Work out the finished part from the listing and answer in its coordinate system (mm). A direction names the side the tool comes from. Round coordinates to 2 decimals unless told otherwise and drop trailing zeros. Loops run counter-clockwise (first coordinate to the right, second up) from the corner with the lowest first, then second, coordinate; pieces in that order, holes last. Notation, with made-up numbers: (58.25, -27.5) -> (114.25, -27.5) arc R16 ccw to (114.25, -3.5) -> close; hole circle Ø4 at (84.5, 71). An arc over 180 degrees is marked (long way). Write item = value, one per line. Start each with the question number.
```python
from build123d import *

# Parameters (mm, degrees)
SKETCH_W        = 69
SKETCH_H        = 43
PAD_DEPTH       = 23
THICKNESS_T     = 1.5
SKETCH001_R     = 1.5
HOLE_DEPTH      = 2.098709
HOLE_TIPS_R     = 1.5
POCKET_DEPTH    = 5
SKETCH003_W     = 8
SKETCH003_H     = 8
PAD001_DEPTH    = 5
SKETCH007_R     = 2.5
POCKET003_DEPTH = 7
SKETCH008_R     = 2.5
POCKET004_DEPTH = 7
SKETCH009_R     = 2.5
POCKET005_DEPTH = 7
SKETCH010_R     = 2.5
POCKET006_DEPTH = 7
POCKET007_DEPTH = 3
FILLET_R        = 1
FILLET001_R     = 1


with BuildPart() as part:
    # Sketch → Pad (new body)
    with BuildSketch(Plane.XY):
        Rectangle(SKETCH_W, SKETCH_H)
    extrude(amount=PAD_DEPTH)

    # Thickness
    thickness_openings = [part.faces().sort_by_distance(p)[0] for p in [
        (0, 0, 23),
    ]]
    offset(amount=THICKNESS_T, openings=thickness_openings)

    # Sketch001 (on Face10 of Thickness) → Hole (cut)
    with BuildSketch(Plane.YZ.offset(36)):
        with Locations((0, 9)):
            Circle(SKETCH001_R)
    extrude(amount=-HOLE_DEPTH, mode=Mode.SUBTRACT)

    # Hole tips → Hole tip 1 section 0
    with BuildSketch(Plane.YZ.offset(33.901291), mode=Mode.PRIVATE) as hole_tip_1_s0:
        with Locations((0, 9)):
            Circle(HOLE_TIPS_R)
    loft([hole_tip_1_s0.sketch, Vertex(33, 0, 9)], mode=Mode.SUBTRACT)

    # Sketch002 (on Face9 of Hole) → Pocket (cut)
    with BuildSketch(Plane(origin=(-36, 0, 0), x_dir=(0, -1, 0), z_dir=(-1, 0, 0))):
        with BuildLine():
            ThreePointArc((-5, 15), (-8, 12), (-5, 9))
            Line((-5, 9), (5, 9))
            ThreePointArc((5, 9), (8, 12), (5, 15))
            Line((-5, 15), (5, 15))
        make_face()
    extrude(amount=-POCKET_DEPTH, mode=Mode.SUBTRACT)

    # Sketch003 (on Face4 of Pocket) → Pad001 (join)
    with BuildSketch(Plane.XY):
        with Locations((-28.95, 15.925)):
            Rectangle(SKETCH003_W, SKETCH003_H)
        with Locations((28.95, 15.925)):
            Rectangle(SKETCH003_W, SKETCH003_H)
        with Locations((-28.95, -15.925)):
            Rectangle(SKETCH003_W, SKETCH003_H)
        with Locations((28.95, -15.925)):
            Rectangle(SKETCH003_W, SKETCH003_H)
    extrude(amount=PAD001_DEPTH)

    # Sketch007 (on Face39 of Pad001) → Pocket003 (cut)
    with BuildSketch(Plane.XY.offset(5)):
        with Locations((-28.95, 15.925)):
            Circle(SKETCH007_R)
    extrude(amount=-POCKET003_DEPTH, mode=Mode.SUBTRACT)

    # Sketch008 (on Face38 of Pocket003) → Pocket004 (cut)
    with BuildSketch(Plane.XY.offset(5)):
        with Locations((28.95, 15.925)):
            Circle(SKETCH008_R)
    extrude(amount=-POCKET004_DEPTH, mode=Mode.SUBTRACT)

    # Sketch009 (on Face37 of Pocket004) → Pocket005 (cut)
    with BuildSketch(Plane.XY.offset(5)):
        with Locations((-28.95, -15.925)):
            Circle(SKETCH009_R)
    extrude(amount=-POCKET005_DEPTH, mode=Mode.SUBTRACT)

    # Sketch010 (on Face36 of Pocket005) → Pocket006 (cut)
    with BuildSketch(Plane.XY.offset(5)):
        with Locations((28.95, -15.925)):
            Circle(SKETCH010_R)
    extrude(amount=-POCKET006_DEPTH, mode=Mode.SUBTRACT)

    # Sketch011 (on Face52 of Pocket006) → Pocket007 (cut)
    with BuildSketch(Plane(origin=(0, 0, -1.5), x_dir=(1, 0, 0), z_dir=(0, 0, -1))):
        Polygon((-25.145774, 17.161068), (-28.95, 19.925), (-32.754226, 17.161068), (-31.301141, 12.688932), (-26.598859, 12.688932), align=None)
        Polygon((26.598859, 12.688932), (31.301141, 12.688932), (32.754226, 17.161068), (28.95, 19.925), (25.145774, 17.161068), align=None)
        Polygon((-26.598859, -12.688932), (-31.301141, -12.688932), (-32.754226, -17.161068), (-28.95, -19.925), (-25.145774, -17.161068), align=None)
        Polygon((26.598859, -12.688932), (25.145774, -17.161068), (28.95, -19.925), (32.754226, -17.161068), (31.301141, -12.688932), align=None)
    extrude(amount=-POCKET007_DEPTH, mode=Mode.SUBTRACT)

    # Fillet
    fillet_edges = [part.edges().sort_by_distance(p)[0] for p in [
        (34.5, 0, 10.5),
    ]]
    fillet(fillet_edges, radius=FILLET_R)

    # Fillet001
    fillet001_edges = [part.edges().sort_by_distance(p)[0] for p in [
        (-36, 0, 0),
        (-36, -21.5, 11.5),
        (-36, 21.5, 11.5),
        (-36, 0, 23),
        (-36, 8, 12),
        (-36, 0, 9),
        (-36, -8, 12),
        (-36, 0, 15),
    ]]
    fillet(fillet001_edges, radius=FILLET001_R)


solid = part.part
```
Item 1: Section B-B (y = -4) is taken. Determine the outline of the cut face in (x, z), then the cut area to 3 significant figures.
Item 2: Find the intervals of material crossed by line 1 along X through (y, z) = (19, 2); line 2 along Y through (x, z) = (-28.95, 2.75) (3 decimals); line 3 along X through (y, z) = (16.5, 15), in increasing order. Write a range as [from, to].
Item 3: The mould has two halves that part along X. Classify faces 4 (the flat face through (0, -21.5, 11)), 5 (the cylindrical face through (35.754, -0.325, 7.536)), 6 (the cylindrical face through (35.57, 22.55, 11.15)): pulls with the +X half, pulls with the -X half, needs draft (parallel to the pull), parting line crosses it, or undercut.
Item 4: Section A-A (z = 19.5) is taken. Determine the outline of the cut face in (x, y).
Item 5: Section C-C (x = -18.5) is taken. Determine the outline of the cut face in (y, z).
Item 6: A flat-ended cylindrical pin translates along its axis: pin 1 (10 mm diameter, centred on x = 24, y = -13, fed in from +Z). Find the tip coordinate at first contact, or state that the pin passes through.
Item 7: A tool of negligible diameter and unlimited length cuts with its end or side. For faces 1 (the cylindrical face through (35.57, 0.3, -1.05)), 2 (the flat face through (-30.879, 18.524, -0.021)), 3 (the flat face through (-29, -19.925, 2)), from which of +Z, -Z, +X, -X, +Y, -Y can it reach the whole face along a straight path? Write none if from no direction.
Worked answers:
q1.outline = (-36, 0) arc R1.5 ccw to (-34.5, -1.5) -> (34.5, -1.5) arc R1.5 ccw to (36, 0) -> (36, 22) arc R1 ccw to (35, 23) -> (34.5, 23) -> (34.5, 0) -> (-34.5, 0) -> (-34.5, 9) -> (-35, 9) arc R1 ccw to (-36, 8) -> close; (-36, 16) arc R1 ccw to (-35, 15) -> (-34.5, 15) -> (-34.5, 23) -> (-35, 23) arc R1 ccw to (-36, 22) -> close
q1.area = 166 mm2
q2.line_1 = [-36, -34.5], [-32.95, -24.95], [24.95, 32.95], [34.5, 36]
q2.line_2 = [-23, -21.5], [-19.925, -18.425], [-13.425, -11.925], [11.925, 13.425], [18.425, 19.925], [21.5, 23]
q2.line_3 = [-36, -34.5], [34.5, 36]
q3.face_4 = undercut
q3.face_5 = needs draft
q3.face_6 = pulls with the +X half
q4.outline = (-36, -21.5) arc R1.5 ccw to (-34.5, -23) -> (34.5, -23) arc R1.5 ccw to (36, -21.5) -> (36, 21.5) arc R1.5 ccw to (34.5, 23) -> (-34.5, 23) arc R1.5 ccw to (-36, 21.5) -> close; hole (-34.5, -21.5) -> (34.5, -21.5) -> (34.5, 21.5) -> (-34.5, 21.5) -> close
q5.outline = (-23, 0) arc R1.5 ccw to (-21.5, -1.5) -> (21.5, -1.5) arc R1.5 ccw to (23, 0) -> (23, 22) arc R1 ccw to (22, 23) -> (21.5, 23) -> (21.5, 0) -> (-21.5, 0) -> (-21.5, 23) -> (-22, 23) arc R1 ccw to (-23, 22) -> close
q6.pin_1 = 5
q7.face_1 = -Z, +X, +Y, -Y
q7.face_2 = -Z
q7.face_3 = +Z
